```python
from build123d import *

# Parameters (mm, degrees)
SKETCH1_W                    = 30
SKETCH1_H                    = 40
BASE_FLANGE1_DEPTH           = 3
EDGE_FLANGE1_STRIP_W         = 13.4732
EDGE_FLANGE1_STRIP_H         = 3
EDGE_FLANGE1_STRIP_CUT_DEPTH = 30
EDGE_FLANGE1_DEPTH           = 30
SKETCH9_R                    = 1.5
CUT_EXTRUDE1_DEPTH           = 10
SKETCH10_R                   = 1.5
CUT_EXTRUDE2_DEPTH           = 10


# Sheet-metal steps are written as plain solids
with BuildPart() as part:
    # Sketch1 → Base-Flange1 (new body)
    with BuildSketch(Plane(origin=(0, 0, 0), x_dir=(1, 0, 0), z_dir=(0, 1, 0))):
        Rectangle(SKETCH1_W, SKETCH1_H)
    extrude(amount=-BASE_FLANGE1_DEPTH)

    # Edge-Flange1 strip (across the edge) → Edge-Flange1 strip cut (cut)
    with BuildSketch(Plane(origin=(15, -3, 20), x_dir=(0, 0, -1), z_dir=(-1, 0, 0))):
        with Locations((-3, -1.5)):
            Rectangle(EDGE_FLANGE1_STRIP_W, EDGE_FLANGE1_STRIP_H)
    extrude(amount=EDGE_FLANGE1_STRIP_CUT_DEPTH, mode=Mode.SUBTRACT)

    # Edge-Flange1 section (across the edge) → Edge-Flange1 (add)
    with BuildSketch(Plane(origin=(15, -3, 20), x_dir=(0, 0, -1), z_dir=(-1, 0, 0))):
        with BuildLine():
            Line((0, 0.7366), (0, 42))
            Line((0, 42), (3, 42))
            Line((3, 42), (3, 0.7366))
            ThreePointArc((3, 0.7366), (3.215745145, 0.215745145), (3.7366, 0))
            Line((3.7366, 0), (3.7366, -3))
            ThreePointArc((3.7366, -3), (1.094424801, -1.905575199), (0, 0.7366))
        make_face()
    extrude(amount=EDGE_FLANGE1_DEPTH)

    # Sketch9 → Cut-Extrude1 (cut)
    with BuildSketch(Plane.XY.offset(20)):
        with Locations((-7.525698427, -21)):
            Circle(SKETCH9_R)
        with Locations((-7.525698427, -37)):
            Circle(SKETCH9_R)
        with Locations(Location((7.525698427, -37, 0), (0, 0, 90))):
            Circle(SKETCH9_R)
        with Locations(Location((7.525698427, -21, 0), (0, 0, 90))):
            Circle(SKETCH9_R)
    extrude(amount=-CUT_EXTRUDE1_DEPTH, mode=Mode.SUBTRACT)

    # Sketch10 → Cut-Extrude2 (cut)
    with BuildSketch(Plane.XZ.offset(3)):
        with Locations(Location((-10.947470665, 11.635125857, 0), (0, 0, 270))):
            Circle(SKETCH10_R)
        with Locations(Location((10.947470665, 11.635125857, 0), (0, 0, 90))):
            Circle(SKETCH10_R)
        with Locations(Location((10.947470665, -11.635125857, 0), (0, 0, 270))):
            Circle(SKETCH10_R)
        with Locations(Location((-10.947470665, -11.635125857, 0), (0, 0, 90))):
            Circle(SKETCH10_R)
    extrude(amount=-CUT_EXTRUDE2_DEPTH, mode=Mode.SUBTRACT)


solid = part.part
```
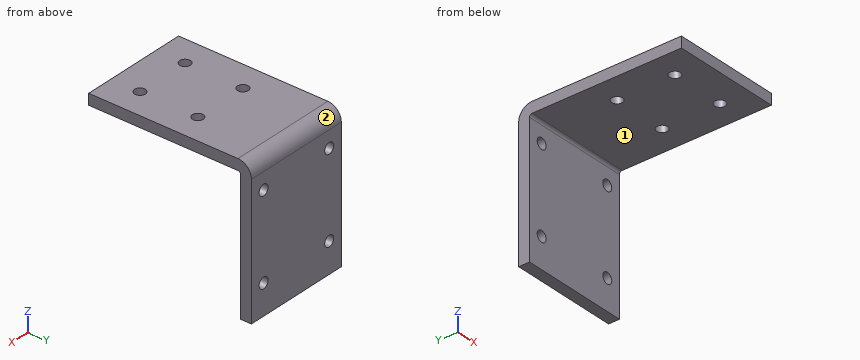
Source: CAD feature listing. Evaluate the final solid. Frame: model axes, mm. Face numbers are marked on the shaded views. A direction names the side the tool comes from. Coordinates: 2 decimals unless noted, no trailing zeros. Loops run counter-clockwise (first coordinate to the right, second up) from the corner with the lowest first, then second, coordinate; pieces in that order, holes last. Notation, with made-up numbers: M 9.25,78.5 L 42.25,78.5 A15 ccw 42.25,89.5 Z; hole C 82.25,1 d3. An arc over 180 degrees is marked long. Put each result on its own line as item: value. Start each with the question number.
1) Reachability of the marked faces 1 and 2 from +Z, -Z, +X, -X, +Y, -Y: full face, straight path, thin tool, end or side. Return the list, or none.
2) Contact query for flat-ended pins moving along their axis: pin 1 Ø10 at (x, z) = (6, 1.5) entering from -Y; pin 2 Ø2.5 at (x, z) = (-10.95, 11.64) entering from +Y; pin 3 Ø1 at (x, y) = (7, -11.5) entering from -Z. Output: stop coordinate, or through.
3) Ray query, L1, parallel to Z at x = -6.5, y = -33; L2, parallel to Y at x = -4.5, z = 9. Return the intervals inside material, ascending. Write a range as from..to.
4) Cut plane A-A on y = -37. Return the cut outline in (x, z).
5) Cut plane D-D on z = 15. Return the cut outline in (x, y), then the cut area to 3 significant figures.
6) Cut plane B-B on x = 2.75. Return the cut outline in (y, z).
7) Cut plane C-C on y = -25.5. Return the cut outline in (x, z).
The answers:
1. face 1: -Z, +X, -X, -Y
1. face 2: +Z, +X, -X, +Y
2. pin 1: stops at y = -3
2. pin 2: passes through
2. pin 3: stops at z = 17
3. L1: z = 17..20
3. L2: y = -3..0
4. outline: M -15,17 L -9.03,17 L -9.03,20 L -15,20 Z; M -6.03,17 L 6.03,17 L 6.03,20 L -6.03,20 Z; M 9.03,17 L 15,17 L 15,20 L 9.03,20 Z
5. outline: M -15,-3 L 15,-3 L 15,0 L -15,0 Z
5. area: 90.0 mm²
6. outline: M -45,17 L -3.74,17 A0.74 cw -3,16.26 L -3,-20 L 0,-20 L 0,16.26 A3.74 ccw -3.74,20 L -45,20 Z
7. outline: M -15,17 L 15,17 L 15,20 L -15,20 Z
